from build123d import *

# Parameters (mm, degrees)
SKETCH1_R           = 96.6
BOSS_EXTRUDE1_DEPTH = 5
SKETCH4_R           = 96.6
SKETCH4_R_2         = 94.6
BOSS_EXTRUDE3_DEPTH = 15
SKETCH5_W           = 189.2
SKETCH5_H           = 13.4
SKETCH5_W_2         = 177
SKETCH5_H_2         = 6.4
BOSS_EXTRUDE4_DEPTH = 15
SKETCH6_R           = 22.5
CUT_EXTRUDE1_DEPTH  = 4
CUT_EXTRUDE2_DEPTH  = 9
BOSS_EXTRUDE6_DEPTH = 15
SKETCH8_R           = 2.175
CUT_EXTRUDE4_DEPTH  = 29
CUT_EXTRUDE9_DEPTH  = 30
FILLET3_R           = 3
SKETCH20_R          = 1.65
CUT_EXTRUDE10_DEPTH = 10
SKETCH24_W          = 25
SKETCH24_H          = 4
BOSS_EXTRUDE8_DEPTH = 35
FILLET2_R           = 10
CUT_EXTRUDE11_DEPTH = 18.8
FILLET4_R           = 6


with BuildPart() as part:
    # Sketch1 → Boss-Extrude1 (new body)
    with BuildSketch(Plane(origin=(0, 0, 0), x_dir=(1, 0, 0), z_dir=(0, 1, 0))):
        with Locations(Location((0, 0, 0), (0, 0, 270))):
            Circle(SKETCH1_R)
    extrude(amount=BOSS_EXTRUDE1_DEPTH)

    # Sketch4 → Boss-Extrude3 (add)
    with BuildSketch(Plane(origin=(0, 5, 0), x_dir=(1, 0, 0), z_dir=(0, 1, 0))):
        with Locations(Location((0, 0, 0), (0, 0, 270))):
            Circle(SKETCH4_R)
        with Locations(Location((0, 0, 0), (0, 0, 270))):
            Circle(SKETCH4_R_2, mode=Mode.SUBTRACT)
    extrude(amount=BOSS_EXTRUDE3_DEPTH)

    # Sketch5 → Boss-Extrude4 (add)
    with BuildSketch(Plane(origin=(0, 5, 0), x_dir=(1, 0, 0), z_dir=(0, 1, 0))):
        with Locations((0, -6.7)):
            Rectangle(SKETCH5_W, SKETCH5_H)
        with Locations((0, -5.2)):
            Rectangle(SKETCH5_W_2, SKETCH5_H_2, mode=Mode.SUBTRACT)
    boss_extrude4 = extrude(amount=BOSS_EXTRUDE4_DEPTH)

    # Mirror1: Boss-Extrude4 across plane
    add(boss_extrude4.mirror(Plane.XY))

    # Sketch6 → Cut-Extrude1 (cut)
    with BuildSketch(Plane.XZ):
        with Locations(Location((0, 0, 0), (0, 0, 270))):
            Circle(SKETCH6_R)
    extrude(amount=-CUT_EXTRUDE1_DEPTH, mode=Mode.SUBTRACT)

    # Sketch7 → Cut-Extrude2 (cut)
    with BuildSketch(Plane(origin=(0, 20, 0), x_dir=(1, 0, 0), z_dir=(0, 1, 0))):
        Polygon((0, -13.4), (-81, -13.4), (-81, -8.4), (0, -8.4), (81, -8.4), (81, -13.4), align=None)
    cut_extrude2 = extrude(amount=-CUT_EXTRUDE2_DEPTH, mode=Mode.SUBTRACT)

    # Mirror2: Cut-Extrude2 across plane
    add(cut_extrude2.mirror(Plane.XY), mode=Mode.SUBTRACT)

    # Sketch10 → Boss-Extrude6 (add)
    with BuildSketch(Plane(origin=(0, 5, 0), x_dir=(1, 0, 0), z_dir=(0, 1, 0))):
        with BuildLine():
            Line((-10, -75.073785704), (-10, -95.073785704))
            Line((-10, -95.073785704), (10, -95.073785704))
            Line((10, -95.073785704), (10, -75.073785704))
            ThreePointArc((10, -75.073785704), (0, -65.073785704), (-10, -75.073785704))
        make_face()
    boss_extrude6 = extrude(amount=BOSS_EXTRUDE6_DEPTH)

    # Mirror3: Boss-Extrude6 across plane
    add(boss_extrude6.mirror(Plane.XY))

    # Sketch8 → Cut-Extrude4 (cut)
    with BuildSketch(Plane.XZ):
        with Locations(Location((-75, 0, 0), (0, 0, 270))):
            Circle(SKETCH8_R)
        with Locations(Location((0, 75, 0), (0, 0, 270))):
            Circle(SKETCH8_R)
        with Locations(Location((75, 0, 0), (0, 0, 270))):
            Circle(SKETCH8_R)
        with Locations(Location((0, -75, 0), (0, 0, 270))):
            Circle(SKETCH8_R)
    extrude(amount=-CUT_EXTRUDE4_DEPTH, mode=Mode.SUBTRACT)

    # Sketch19 → Cut-Extrude9 (cut)
    with BuildSketch(Plane(origin=(0, 5, 0), x_dir=(1, 0, 0), z_dir=(0, 1, 0))):
        with BuildLine():
            Line((-55.725373322, -31.475113472), (55.725373322, -31.475113472))
            ThreePointArc((55.725373322, -31.475113472), (0, -64), (-55.725373322, -31.475113472))
        make_face()
    cut_extrude9 = extrude(amount=-CUT_EXTRUDE9_DEPTH, mode=Mode.SUBTRACT)

    # Mirror4: Cut-Extrude9 across plane
    add(cut_extrude9.mirror(Plane.XY), mode=Mode.SUBTRACT)

    # Fillet3
    fillet3_edges = [part.edges().sort_by_distance(p)[0] for p in [
        (81, 20, -10.9),
        (-81, 20, -10.9),
        (81, 11, -10.9),
        (-81, 11, -10.9),
        (-81, 11, 10.9),
        (81, 11, 10.9),
        (81, 20, 10.9),
        (-81, 20, 10.9),
    ]]
    fillet(fillet3_edges, radius=FILLET3_R)

    # Sketch20 → Cut-Extrude10 (cut)
    with BuildSketch(Plane.XZ):
        with Locations(Location((-64.346717088, 64.346717088, 0), (0, 0, 270))):
            Circle(SKETCH20_R)
        with Locations(Location((64.346717088, 64.346717088, 0), (0, 0, 270))):
            Circle(SKETCH20_R)
        with Locations(Location((64.346717088, -64.346717088, 0), (0, 0, 270))):
            Circle(SKETCH20_R)
        with Locations(Location((-64.346717088, -64.346717088, 0), (0, 0, 270))):
            Circle(SKETCH20_R)
    extrude(amount=-CUT_EXTRUDE10_DEPTH, mode=Mode.SUBTRACT)

    # Sketch24 → Boss-Extrude8 (add)
    with BuildSketch(Plane(origin=(0, 20, 0), x_dir=(1, 0, 0), z_dir=(0, 1, 0))):
        Rectangle(SKETCH24_W, SKETCH24_H)
    extrude(amount=BOSS_EXTRUDE8_DEPTH)

    # Fillet2
    fillet2_edges = [part.edges().sort_by_distance(p)[0] for p in [
        (12.5, 20, 0),
        (-12.5, 20, 0),
        (12.5, 55, 0),
        (-12.5, 55, 0),
    ]]
    fillet(fillet2_edges, radius=FILLET2_R)

    # Sketch25 → Cut-Extrude11 (cut)
    with BuildSketch(Plane(origin=(0, 20, 0), x_dir=(1, 0, 0), z_dir=(0, 1, 0))):
        Polygon((70.843078062, 0), (72.921539031, -3.6), (77.078460969, -3.6), (79.156921938, 0), (77.078460969, 3.6), (72.921539031, 3.6), align=None)
        Polygon((-70.843078062, 0), (-72.921539031, 3.6), (-77.078460969, 3.6), (-79.156921938, 0), (-77.078460969, -3.6), (-72.921539031, -3.6), align=None)
    extrude(amount=-CUT_EXTRUDE11_DEPTH, mode=Mode.SUBTRACT)

    # Fillet4
    fillet4_edges = [part.edges().sort_by_distance(p)[0] for p in [
        (0, 5, 13.4),
        (93.646142473, 12.5, 13.4),
        (-93.646142473, 12.5, 13.4),
        (93.646142473, 12.5, -13.4),
        (-93.646142473, 12.5, -13.4),
        (0, 5, -13.4),
    ]]
    fillet(fillet4_edges, radius=FILLET4_R - 0.0001)  # a hair under: the kernel refuses the full size


solid = part.part
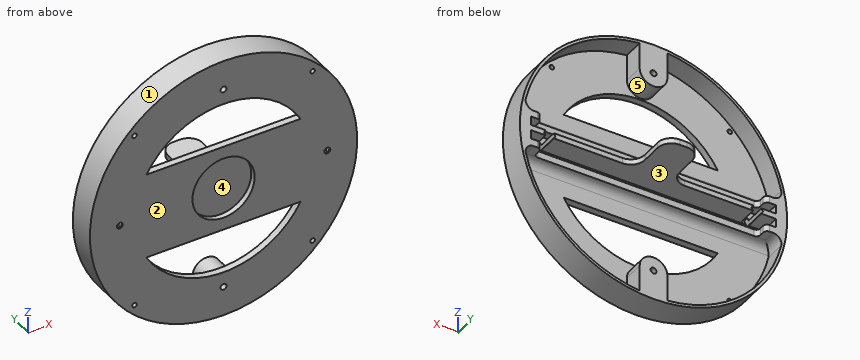
Model file for the job. Use its own axes, mm. Face numbers are marked on the shaded views. A direction names the side the tool comes from. Round coordinates to 2 decimals unless told otherwise and drop trailing zeros. Loops run counter-clockwise (first coordinate to the right, second up) from the corner with the lowest first, then second, coordinate; pieces in that order, holes last.
1. Tool access for the marked faces 4 and 5: list every direction of +Z, -Z, +X, -X, +Y, -Y with a clear straight run to the whole face (end or side of a thin tool).
Check values:
face 4: -Y
face 5: +Y
2. Band-saw the part on A-A, the plane z = 39. List the corners of the cut face in (x, y).
Check values:
outline: (-88.38, 0) - (-50.74, 0) - (-50.74, 5) - (-86.19, 5) - (-86.19, 20) - (-88.38, 20) - close; (50.74, 0) - (88.38, 0) - (88.38, 20) - (86.19, 20) - (86.19, 5) - (50.74, 5) - close
3. Mould opens along Z. For the marked faces 1, 2 and 3 say: +Z half, -Z half, draft (parallel to the pull), parting line (faces both ways), or undercut.
Check values:
face 1: parting line
face 2: draft
face 3: undercut
4. Wall check: probe 1 along X at (y, z) = (10.5, -75) (3 decimals); probe 2 along Y at (x, z) = (-73, 47.5); probe 3 along Z at (x, y) = (25.5, 13). Give the ranges that are in metal, low to high.
Check values:
probe 1: x = -60.882 to -57.656, -10 to -2.175, 2.175 to 10, 57.656 to 60.882
probe 2: y = 0 to 5
probe 3: z = -93.17 to -91.1, -2 to 2, 91.1 to 93.17
5. Drop flat-ended pins along their axis: P1, Ø2, axis at x = -66, z = -48.5, coming from the -Y side; P2, Ø1.2, axis at y = 35, z = 0, coming from the -X side; P3, Ø1.5, axis at x = -19.5, z = -7, coming from the -Y side; P4, Ø4.5, axis at x = -64.35, z = 64.35, coming from the +Y side. Give the stop position or say it passes through.
Check values:
P1: stops at y = 0
P2: stops at x = -12.5
P3: stops at y = 4
P4: stops at y = 5
6. Band-saw the part on C-C, the plane z = -34. List the corners of the cut face in (x, y).
Check values:
outline: (-90.42, 0) - (-54.22, 0) - (-54.22, 5) - (-88.28, 5) - (-88.28, 20) - (-90.42, 20) - close; (54.22, 0) - (90.42, 0) - (90.42, 20) - (88.28, 20) - (88.28, 5) - (54.22, 5) - close
7. Band-saw the part on B-B, the plane x = -36.5. Count the separate pieces of the cut face and the enclosed holes in it, and give its area (3 significant figures).
Check values:
separate pieces: 3
enclosed holes: 0
area: 884 mm2
8. Band-saw the part on D-D, the plane y = 25.5. List the corners of the cut face in (x, z).
Check values:
outline: (-13.57, -2) - (13.57, -2) - (13.57, 2) - (-13.57, 2) - close
